Design review of the part built by this model. Coordinates are the model's own, in mm. A direction names the side the tool comes from. Coordinates: 2 decimals unless noted, no trailing zeros. Write each loop counter-clockwise with the first axis right and the second up, starting at its lowest first coordinate (ties: lowest second). Pieces come first, ordered by that corner, then holes. Notation, with made-up numbers: (-9.75, -37) -> (-1.75, -37) arc R16 cw to (-1.75, -13) -> close; hole circle Ø1 at (24, 47.5). An arc over 180 degrees is marked (long way). Answer in a Markdown table with one row per item. Add a question column.
Item 1: Take a section at A-A, the plane y = 5. Write out the cut boundary in (x, z), and give its area (3 significant figures).
Item 2: To check wall thickness, follow line 1 (X direction, y = 5.5, z = 0); line 2 (X direction, y = 14.7, z = 0); line 3 (Y direction, x = 3, z = -1.5). State the ranges of each line that lie inside material, in increasing order.
Item 3: Clearance check with flat-ended pins moving along their axes: P1, Ø3.5, axis at x = 1.5, z = 0, coming from the -Y side; P2, Ø4, axis at x = -0.5, y = 10, coming from the +Z side; P3, Ø4, axis at x = 9, y = 12.5, coming from the +Z side. State where each tip first meets the part, or that it passes through.
Item 4: Draft analysis for pull direction Z (two halves, no side actions). For faces 6 (the face through (-13.5, 9.1, 0)), 7 (the face through (-8.45, 9.08, -10.53)), 8 (the face through (12.18, 9.08, 5.82)), 9 (the face through (7, 15, 9)), state which applies: released by +Z, released by -Z, zero draft, split by the parting line, or undercut.
Item 5: For faces 1 (the face through (9, 9, 12)), 2 (the face through (9, 9, -12)), 3 (the face through (-13.49, 9.08, -6.56)), 4 (the face through (3.17, 3.4, -13.74)), 5 (the face through (12.69, 3.4, 6.15)), list the 3-axis set-ups (+Z, -Z, +X, -X, +Y, -Y) from which the entire face can be reached by the end or side of a thin tool; tool diameter is ignored.
Item 6: Take a section at D-D, the plane x = 0. Write out the cut boundary in (y, z), and give its area (3 significant figures).
Item 7: Take a section at B-B, the plane z = 0. Write out the cut boundary in (x, y), and give its area (3 significant figures).
Item 8: Take a section at C-C, the plane y = 13.5. Write out the cut boundary in (x, z), and give its area (3 significant figures).
from build123d import *

# Parameters (mm, degrees)
SKETCH2_R          = 3.6
CUT_EXTRUDE1_DEPTH = 10
SKETCH3_R          = 4
CUT_EXTRUDE2_DEPTH = 11
CHAMFER1_SIZE      = 1.5


with BuildPart() as part:
    # Sketch1 → Revolve1 (revolve)
    with BuildSketch(Plane(origin=(0, 0, 0), x_dir=(0, 0, -1), z_dir=(1, 0, 0)), mode=Mode.PRIVATE) as revolve1_sk:
        Polygon((0, 0), (-16.5, 0), (-16.5, 3), (-15, 3), (-15, 15), (-11, 15), (-11, 14.355733533), (0, 14.355733533), align=None)
    revolve(revolve1_sk.sketch.rotate(Axis((0, 0, 0), (0, 1, 0)), 180), axis=Axis((0, 0, 0), (0, 1, 0)))

    # Sketch2 → Cut-Extrude1 (cut)
    with BuildSketch(Plane.XZ):
        with Locations(Location((0, 0, 0), (0, 0, 270))):
            Circle(SKETCH2_R)
    extrude(amount=-CUT_EXTRUDE1_DEPTH, mode=Mode.SUBTRACT)

    # Sketch3 → Cut-Extrude2 (cut)
    with BuildSketch(Plane(origin=(0, 15, 0), x_dir=(1, 0, 0), z_dir=(0, 1, 0))):
        with Locations((-17.5, 0)):
            Circle(SKETCH3_R)
        with Locations((-10.911071533, 13.682050943)):
            Circle(SKETCH3_R)
        with Locations((3.894116344, 17.061238463)):
            Circle(SKETCH3_R)
        with Locations((15.766955188, 7.592965435)):
            Circle(SKETCH3_R)
        with Locations((15.766955188, -7.592965435)):
            Circle(SKETCH3_R)
        with Locations((3.894116344, -17.061238463)):
            Circle(SKETCH3_R)
        with Locations((-10.911071533, -13.682050943)):
            Circle(SKETCH3_R)
    extrude(amount=-CUT_EXTRUDE2_DEPTH, mode=Mode.SUBTRACT)

    # Chamfer1
    # the kernel refuses this chamfer: 1.5 mm, written as the material it takes off along each edge
    with BuildSketch(Plane(origin=(0, 4, 0), x_dir=(-0.22388554303077474, 0, 0.974615443968448), z_dir=(-0.974615443968448, 0, -0.22388554303077474))) as chamfer1_piece_1_section:
        Polygon((15, -CHAMFER1_SIZE), (15 - CHAMFER1_SIZE, 0), (15, 0), align=None)
    chamfer1_piece_1 = revolve(axis=Axis((0, 4, 0), (0, 1, 0)), revolution_arc=51.588991206, mode=Mode.PRIVATE)
    chamfer1_piece_1 = split(chamfer1_piece_1, bisect_by=Plane(origin=(3.219301063, 3, 14.104691916), z_dir=(0, 1, 0)), keep=Keep.TOP, mode=Mode.PRIVATE)
    chamfer1_piece_1 = chamfer1_piece_1 & Plane(origin=(3.894116344, 3.575453248, 17.061238463), x_dir=(1, 0, 0), z_dir=(0, 1, 0)) * Cylinder(4, 60, mode=Mode.PRIVATE)
    add(chamfer1_piece_1, mode=Mode.SUBTRACT)
    with BuildSketch(Plane(origin=(0, 4, 0), x_dir=(-0.9015753902573829, 0, 0.43262202403743605), z_dir=(-0.43262202403743605, 0, -0.9015753902573829))) as chamfer1_piece_2_section:
        Polygon((15, -CHAMFER1_SIZE), (15 - CHAMFER1_SIZE, 0), (15, 0), align=None)
    chamfer1_piece_2 = revolve(axis=Axis((0, 4, 0), (0, 1, 0)), revolution_arc=51.588991206, mode=Mode.PRIVATE)
    chamfer1_piece_2 = split(chamfer1_piece_2, bisect_by=Plane(origin=(-9.020290662, 3, 11.311082492), z_dir=(0, 1, 0)), keep=Keep.TOP, mode=Mode.PRIVATE)
    chamfer1_piece_2 = chamfer1_piece_2 & Plane(origin=(-10.911071533, 3.575453183, 13.682050943), x_dir=(1, 0, 0), z_dir=(0, 1, 0)) * Cylinder(4, 60, mode=Mode.PRIVATE)
    add(chamfer1_piece_2, mode=Mode.SUBTRACT)
    with BuildSketch(Plane(origin=(0, 4, 0), x_dir=(-0.9003605798337992, 0, -0.4351446038747863), z_dir=(0.4351446038747863, 0, -0.9003605798337992))) as chamfer1_piece_3_section:
        Polygon((15, -CHAMFER1_SIZE), (15 - CHAMFER1_SIZE, 0), (15, 0), align=None)
    chamfer1_piece_3 = revolve(axis=Axis((0, 4, 0), (0, 1, 0)), revolution_arc=51.588991206, mode=Mode.PRIVATE)
    chamfer1_piece_3 = split(chamfer1_piece_3, bisect_by=Plane(origin=(-14.467418648, 3, -5.57e-07), z_dir=(0, 1, 0)), keep=Keep.TOP, mode=Mode.PRIVATE)
    chamfer1_piece_3 = chamfer1_piece_3 & Plane(origin=(-17.5, 3.575453666, 0), x_dir=(1, 0, 0), z_dir=(0, 1, 0)) * Cylinder(4, 60, mode=Mode.PRIVATE)
    add(chamfer1_piece_3, mode=Mode.SUBTRACT)
    with BuildSketch(Plane(origin=(0, 4, 0), x_dir=(-0.2211558887866005, 0, -0.9752384697370221), z_dir=(0.9752384697370221, 0, -0.2211558887866005))) as chamfer1_piece_4_section:
        Polygon((15, -CHAMFER1_SIZE), (15 - CHAMFER1_SIZE, 0), (15, 0), align=None)
    chamfer1_piece_4 = revolve(axis=Axis((0, 4, 0), (0, 1, 0)), revolution_arc=51.588991206, mode=Mode.PRIVATE)
    chamfer1_piece_4 = split(chamfer1_piece_4, bisect_by=Plane(origin=(-9.020286489, 3, -11.311086109), z_dir=(0, 1, 0)), keep=Keep.TOP, mode=Mode.PRIVATE)
    chamfer1_piece_4 = chamfer1_piece_4 & Plane(origin=(-10.911071533, 3.575453389, -13.682050943), x_dir=(1, 0, 0), z_dir=(0, 1, 0)) * Cylinder(4, 60, mode=Mode.PRIVATE)
    add(chamfer1_piece_4, mode=Mode.SUBTRACT)
    with BuildSketch(Plane(origin=(0, 4, 0), x_dir=(0.6245836972749009, 0, -0.7809578766479117), z_dir=(0.7809578766479117, 0, 0.6245836972749009))) as chamfer1_piece_5_section:
        Polygon((15, -CHAMFER1_SIZE), (15 - CHAMFER1_SIZE, 0), (15, 0), align=None)
    chamfer1_piece_5 = revolve(axis=Axis((0, 4, 0), (0, 1, 0)), revolution_arc=51.588991206, mode=Mode.PRIVATE)
    chamfer1_piece_5 = split(chamfer1_piece_5, bisect_by=Plane(origin=(3.219306774, 3, -14.104690845), z_dir=(0, 1, 0)), keep=Keep.TOP, mode=Mode.PRIVATE)
    chamfer1_piece_5 = chamfer1_piece_5 & Plane(origin=(3.894116344, 3.575453353, -17.061238463), x_dir=(1, 0, 0), z_dir=(0, 1, 0)) * Cylinder(4, 60, mode=Mode.PRIVATE)
    add(chamfer1_piece_5, mode=Mode.SUBTRACT)
    with BuildSketch(Plane(origin=(0, 4, 0), x_dir=(0.9999990201028447, 0, 0.001399926194576086), z_dir=(-0.001399926194576086, 0, 0.9999990201028447))) as chamfer1_piece_6_section:
        Polygon((15, -CHAMFER1_SIZE), (15 - CHAMFER1_SIZE, 0), (15, 0), align=None)
    chamfer1_piece_6 = revolve(axis=Axis((0, 4, 0), (0, 1, 0)), revolution_arc=51.588991206, mode=Mode.PRIVATE)
    chamfer1_piece_6 = split(chamfer1_piece_6, bisect_by=Plane(origin=(13.034696257, 3, -6.2771755), z_dir=(0, 1, 0)), keep=Keep.TOP, mode=Mode.PRIVATE)
    chamfer1_piece_6 = chamfer1_piece_6 & Plane(origin=(15.766955188, 3.575453245, -7.592965435), x_dir=(1, 0, 0), z_dir=(0, 1, 0)) * Cylinder(4, 60, mode=Mode.PRIVATE)
    add(chamfer1_piece_6, mode=Mode.SUBTRACT)
    with BuildSketch(Plane(origin=(0, 4, 0), x_dir=(0.622394684530797, 0, 0.782703556059259), z_dir=(-0.782703556059259, 0, 0.622394684530797))) as chamfer1_piece_7_section:
        Polygon((15, -CHAMFER1_SIZE), (15 - CHAMFER1_SIZE, 0), (15, 0), align=None)
    chamfer1_piece_7 = revolve(axis=Axis((0, 4, 0), (0, 1, 0)), revolution_arc=51.588991206, mode=Mode.PRIVATE)
    chamfer1_piece_7 = split(chamfer1_piece_7, bisect_by=Plane(origin=(13.03469369, 3, 6.277180857), z_dir=(0, 1, 0)), keep=Keep.TOP, mode=Mode.PRIVATE)
    chamfer1_piece_7 = chamfer1_piece_7 & Plane(origin=(15.766955188, 3.575453554, 7.592965435), x_dir=(1, 0, 0), z_dir=(0, 1, 0)) * Cylinder(4, 61, mode=Mode.PRIVATE)
    add(chamfer1_piece_7, mode=Mode.SUBTRACT)


solid = part.part
Answers:
| question | item | result |
|---|---|---|
| 1 | outline | (-14.72, -2.88) arc R15 ccw to (-11.43, -9.72) arc R4 cw to (-6.93, -13.3) arc R15 ccw to (0.47, -14.99) arc R4 cw to (6.08, -13.71) arc R15 ccw to (12.02, -8.98) arc R4 cw to (14.51, -3.79) arc R15 ccw to (14.51, 3.79) arc R4 cw to (12.02, 8.98) arc R15 ccw to (6.08, 13.71) arc R4 cw to (0.47, 14.99) arc R15 ccw to (-6.93, 13.3) arc R4 cw to (-11.43, 9.72) arc R15 ccw to (-14.72, 2.88) arc R4 cw to start; hole circle Ø7.2 at (0, 0) |
| 1 | area | 625 mm^2 |
| 2 | line 1 | x = -13.5 to -3.6, 3.6 to 15 |
| 2 | line 2 | x = -13.5 to -11, 11 to 15 |
| 2 | line 3 | y = 10 to 14.36 |
| 3 | P1 | stops at y = 10 |
| 3 | P2 | stops at z = 15 |
| 3 | P3 | stops at z = 13.27 |
| 4 | face 6 | undercut |
| 4 | face 7 | released by -Z |
| 4 | face 8 | undercut |
| 4 | face 9 | zero draft |
| 5 | face 1 | +Z, +X, +Y |
| 5 | face 2 | -Z, +X, +Y |
| 5 | face 3 | -Z, -X, +Y |
| 5 | face 4 | -Z, +Y |
| 5 | face 5 | +X, +Y |
| 6 | outline | (0, -16.5) -> (3, -16.5) -> (3, -15) -> (15, -15) -> (15, -11) -> (14.36, -11) -> (14.36, 11) -> (15, 11) -> (15, 15) -> (3, 15) -> (3, 16.5) -> (0, 16.5) -> (0, 3.6) -> (10, 3.6) -> (10, -3.6) -> (0, -3.6) -> close |
| 6 | area | 373 mm^2 |
| 7 | outline | (-16.5, 0) -> (-3.6, 0) -> (-3.6, 10) -> (3.6, 10) -> (3.6, 0) -> (16.5, 0) -> (16.5, 3) -> (15, 3) -> (15, 15) -> (11, 15) -> (11, 14.36) -> (-11, 14.36) -> (-11, 15) -> (-13.5, 15) -> (-13.5, 4) -> (-14.5, 3) -> (-16.5, 3) -> close |
| 7 | area | 355 mm^2 |
| 8 | outline | (-14.72, -2.88) arc R15 ccw to (-11.43, -9.72) arc R4 cw to (-6.93, -13.3) arc R15 ccw to (0.47, -14.99) arc R4 cw to (6.08, -13.71) arc R15 ccw to (12.02, -8.98) arc R4 cw to (14.51, -3.79) arc R15 ccw to (14.51, 3.79) arc R4 cw to (12.02, 8.98) arc R15 ccw to (6.08, 13.71) arc R4 cw to (0.47, 14.99) arc R15 ccw to (-6.93, 13.3) arc R4 cw to (-11.43, 9.72) arc R15 ccw to (-14.72, 2.88) arc R4 cw to start |
| 8 | area | 665 mm^2 |
